```python
from build123d import *

# Parameters (mm, degrees)
F1_DEPTH      = 100
F2_W          = 3
F2_H          = 1.333333
F2_H_2        = 1.333334
F3_DEPTH      = 1
F4_W          = 23.250002
F4_H          = 62
F5_DEPTH      = 1.001
F5_DEPTH_BACK = 11.001


with BuildPart() as f1:
    # F0 (on Front) → F1 (new body)
    with BuildSketch(Plane.XZ):
        Polygon((3, 0), (0, 0), (0, -1), (2, -1), (2, -11), (11.5, -11), (11.5, -1), (13.5, -1), (13.5, 0), (10.5, 0), (10.5, -10), (3, -10), align=None)
    extrude(amount=F1_DEPTH)

    # F2 (on face) → F3 (join)
    with BuildSketch(Plane.XY):
        with Locations((1.5, -0.666666)):
            Rectangle(F2_W, F2_H)
        with Locations((12, -0.666666)):
            Rectangle(F2_W, F2_H)
        with Locations((1.5, -13)):
            Rectangle(F2_W, F2_H_2)
        with Locations((12, -13)):
            Rectangle(F2_W, F2_H_2)
        with Locations((1.5, -25.333334)):
            Rectangle(F2_W, F2_H)
        with Locations((12, -25.333334)):
            Rectangle(F2_W, F2_H)
        with Locations((1.5, -37.666666)):
            Rectangle(F2_W, F2_H)
        with Locations((12, -37.666666)):
            Rectangle(F2_W, F2_H)
        with Locations((1.5, -50)):
            Rectangle(F2_W, F2_H_2)
        with Locations((12, -50)):
            Rectangle(F2_W, F2_H_2)
        with Locations((1.5, -62.333333)):
            Rectangle(F2_W, F2_H)
        with Locations((12, -62.333333)):
            Rectangle(F2_W, F2_H)
        with Locations((1.5, -74.666666)):
            Rectangle(F2_W, F2_H)
        with Locations((12, -74.666666)):
            Rectangle(F2_W, F2_H)
        with Locations((1.5, -87)):
            Rectangle(F2_W, F2_H_2)
        with Locations((12, -87)):
            Rectangle(F2_W, F2_H_2)
        with Locations((1.5, -99.333333)):
            Rectangle(F2_W, F2_H)
        with Locations((12, -99.333333)):
            Rectangle(F2_W, F2_H)
    extrude(amount=F3_DEPTH)

    # F4 (on Top) → F5 (cut, two sides)
    with BuildSketch(Plane.XY) as f5_sk:
        with Locations((11.625001, -31)):
            Rectangle(F4_W, F4_H)
    extrude(amount=F5_DEPTH, mode=Mode.SUBTRACT)
    extrude(f5_sk.sketch, amount=-F5_DEPTH_BACK, mode=Mode.SUBTRACT)


solid = f1.part
```
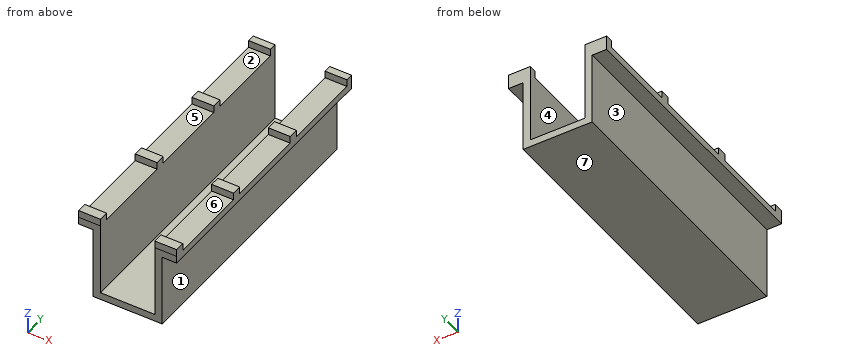
The listing builds one solid part. Answer for the finished solid, in the listing's coordinates (mm). Face numbers are marked on the shaded views. A direction names the side the tool comes from. Coordinates: 2 decimals unless noted, no trailing zeros. Order: outer loops, then holes, each group sorted by start corner. A loop starts at its lowest first (then second) coordinate and runs counter-clockwise, first axis right, second up. Notation, with made-up numbers: M -29.75,89.5 L -4.75,89.5 A9 cw -4.75,105.5 Z; hole C 48.5,37 d2. An arc over 180 degrees is marked long. Answer as a JSON object with one key per item and string values. Group by question number.
1. Section B-B on x = 1 is taken. Write down the section's boundary in (y, z).
2. Flat-ended cylindrical pins translate along their axes: P1, Ø3.5, axis at y = -89, z = -3, coming from the -X side; P2, Ø5, axis at x = 1.5, y = -88.5, coming from the +Z side; P3, Ø1.5, axis at x = 11.5, y = -79.5, coming from the +Z side; P4, Ø2, axis at x = 8, z = -4, coming from the +Y side. Find the tip coordinate at first contact, or state that the pin passes through.
3. Section A-A on z = -6 is taken. Write down the section's boundary in (x, y), then the cut area to 3 significant figures.
4. A tool of negligible diameter and unlimited length cuts with its end or side. For the marked faces 1, 2, 3 and 4, from which of +Z, -Z, +X, -X, +Y, -Y can it reach the whole face along a straight path? Write none if from no direction.
5. Straight lines are drawn through the part: line 1 (X direction, y = -82, z = -3.25); line 2 (X direction, y = -89, z = -0.5); line 3 (Z direction, x = 10.25, y = -75). For each, find the intervals that lie inside material, in ascending order.
6. Section C-C on y = -77.5 is taken. Write down the section's boundary in (x, z), then the cut area to 3 significant figures.
7. Section D-D on x = 6.5 is taken. Write down the section's boundary in (y, z).
8. Determine the mould class of the marked faces 5, 6 and 7 for opening direction Y: released by +Y, released by -Y, zero draft, split by the parting line, or undercut.
Values follow:
{
 "1": {"outline": "M -100,-1 L -62,-1 L -62,1 L -63,1 L -63,0 L -74,0 L -74,1 L -75.33,1 L -75.33,0 L -86.33,0 L -86.33,1 L -87.67,1 L -87.67,0 L -98.67,0 L -98.67,1 L -100,1 Z"},
 "2": {"P1": "x = 2", "P2": "z = 1", "P3": "z = 0", "P4": "through"},
 "3": {"outline": "M 2,-100 L 3,-100 L 3,-62 L 2,-62 Z; M 10.5,-100 L 11.5,-100 L 11.5,-62 L 10.5,-62 Z", "area": "76.0 mm2"},
 "4": {"face 1": "-Z, +X, +Y, -Y", "face 2": "+Z, +X, -X", "face 3": "-Z, -X, +Y, -Y", "face 4": "+Z, +Y, -Y"},
 "5": {"line 1": "2 to 3, 10.5 to 11.5", "line 2": "0 to 3, 10.5 to 13.5", "line 3": "-11 to -10"},
 "6": {"outline": "M 0,-1 L 2,-1 L 2,-11 L 11.5,-11 L 11.5,-1 L 13.5,-1 L 13.5,0 L 10.5,0 L 10.5,-10 L 3,-10 L 3,0 L 0,0 Z", "area": "33.5 mm2"},
 "7": {"outline": "M -100,-11 L -62,-11 L -62,-10 L -100,-10 Z"},
 "8": {"face 5": "undercut", "face 6": "undercut", "face 7": "zero draft"}
}
